Source: CAD feature listing. Evaluate the final solid. Frame: model axes, mm. Face numbers are marked on the shaded views. A direction names the side the tool comes from. Round coordinates to 2 decimals unless told otherwise and drop trailing zeros. Order: outer loops, then holes, each group sorted by start corner. A loop starts at its lowest first (then second) coordinate and runs counter-clockwise, first axis right, second up. Notation, with made-up numbers: (-37.75, -12) - (10.25, -12) arc R22 cw to (10.25, 8) - close; hole circle Ø2 at (-39.75, 34). An arc over 180 degrees is marked (long way). Use one line per item in the form item = value. Start each with the question number.
Q1. Ray query, line 1 (Z direction, x = -6, y = -16); line 2 (Z direction, x = -4.5, y = -15.5); line 3 (X direction, y = -16.5, z = 16). Return the intervals inside material, ascending. Write a range as [from, to].
Q2. Draft query along Z for the marked faces 4, 5 and 6. Return one class per face: released by +Z, released by -Z, zero draft, split by the parting line, or undercut.
Q3. Cut plane B-B, the plane x = -11.5. Return the cut outline in (y, z), and give its area (3 significant figures).
Q4. Cut plane C-C, the plane z = 12. Return the cut outline in (x, y), and give its area (3 significant figures).
Q5. Cut plane D-D, the plane y = 6. Return the cut outline in (x, z).
Q6. Cut plane A-A, the plane y = -10. Return the cut outline in (x, z).
Q7. Set-up query: the marked faces 1, 2 and 3. Return all of +Z, -Z, +X, -X, +Y, -Y with unobstructed straight access to the full face (end or side cutting, diameter ignored); none if empty.
Q8. Pin query (flat end, axial travel): pin 1 Ø1 at (y, z) = (-0.5, -10.5) entering from +X; pin 2 Ø1.5 at (y, z) = (-0.5, -18) entering from +X; pin 3 Ø1.5 at (x, y) = (-12.5, 5) entering from +Z; pin 4 Ø3 at (x, y) = (-14.5, -11) entering from +Z. Return the tip coordinate at first contact, or that it passes through.
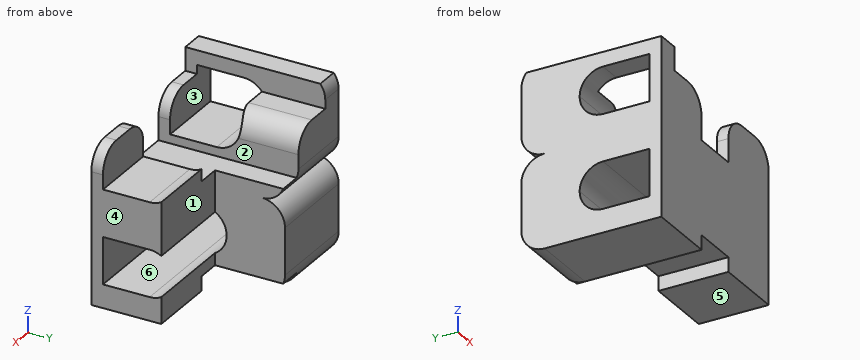
from build123d import *

# Parameters (mm, degrees)
F3_DEPTH = 25
F4_DEPTH = 25
F2_W     = 5
F2_H     = 5
F2_W_2   = 10
F2_H_2   = 20
F5_DEPTH = 25


with BuildPart() as f3:
    # F0 (on Top) → F3 (new body, symmetric)
    with BuildSketch(Plane.XY):
        Polygon((0, 20), (-20, 20), (-20, -20), (20, -20), (20, -5), (0, -5), align=None)
    extrude(amount=F3_DEPTH, both=True)

    # F1 (on Right) → F4 (intersect, symmetric)
    with BuildSketch(Plane.YZ):
        with BuildLine():
            Line((5, 20), (-20, 20))
            Line((-20, 20), (-20, -20))
            Line((-20, -20), (5, -20))
            ThreePointArc((5, -20), (8.535534, -18.535534), (10, -15))
            Line((10, -15), (10, -5))
            ThreePointArc((10, -5), (8.535534, -1.464466), (5, 0))
            ThreePointArc((5, 0), (8.535534, 1.464466), (10, 5))
            Line((10, 5), (10, 15))
            ThreePointArc((10, 15), (8.535534, 18.535534), (5, 20))
        make_face()
        with BuildLine():
            Line((-17.5, -5), (-7.5, -5))
            ThreePointArc((-7.5, -5), (-3.964466, -6.464466), (-2.5, -10))
            ThreePointArc((-2.5, -10), (-3.964466, -13.535534), (-7.5, -15))
            Line((-7.5, -15), (-17.5, -15))
            Line((-17.5, -15), (-17.5, -5))
        make_face(mode=Mode.SUBTRACT)
        with BuildLine():
            Line((-17.5, 15), (-7.5, 15))
            ThreePointArc((-7.5, 15), (-3.964466, 13.535534), (-2.5, 10))
            ThreePointArc((-2.5, 10), (-3.964466, 6.464466), (-7.5, 5))
            Line((-7.5, 5), (-17.5, 5))
            Line((-17.5, 5), (-17.5, 15))
        make_face(mode=Mode.SUBTRACT)
    extrude(amount=F4_DEPTH, both=True, mode=Mode.INTERSECT)

    # F2 (on Front) → F5 (intersect, symmetric)
    with BuildSketch(Plane.XZ):
        with Locations((-17.5, 15.590909)):
            Rectangle(F2_W, F2_H)
        with BuildLine():
            Line((-15, 13.090909), (-20, 13.090909))
            Line((-20, 13.090909), (-20, -21.909091))
            Line((-20, -21.909091), (-5, -21.909091))
            Line((-5, -21.909091), (-5, -16.909091))
            Line((-5, -16.909091), (-5, 3.090909))
            Line((-5, 3.090909), (-5, 8.090909))
            ThreePointArc((-5, 8.090909), (-6.464466, 11.626443), (-10, 13.090909))
            Line((-10, 13.090909), (-15, 13.090909))
        make_face()
        with Locations((0, -6.909091)):
            Rectangle(F2_W_2, F2_H_2)
        with BuildLine():
            Line((5, 3.090909), (5, -16.909091))
            Line((5, -16.909091), (5, -21.909091))
            Line((5, -21.909091), (20, -21.909091))
            Line((20, -21.909091), (20, 8.090909))
            ThreePointArc((20, 8.090909), (18.535534, 11.626443), (15, 13.090909))
            Line((15, 13.090909), (10, 13.090909))
            ThreePointArc((10, 13.090909), (6.464466, 11.626443), (5, 8.090909))
            Line((5, 8.090909), (5, 3.090909))
        make_face()
    extrude(amount=F5_DEPTH, both=True, mode=Mode.INTERSECT)


solid = f3.part
Completed:
q1.line_1 = [-20, -15], [-5, 5]
q1.line_2 = [-16.91, -15], [-5, 3.09]
q1.line_3 = [-20, -15]
q2.face_4 = zero draft
q2.face_5 = released by -Z
q2.face_6 = undercut
q3.outline = (-20, -20) - (5, -20) arc R5 ccw to (10, -15) - (10, -5) arc R5 ccw to (5, 0) arc R5 ccw to (10, 5) - (10, 13.09) - (-3.57, 13.09) arc R5 cw to (-7.5, 5) - (-17.5, 5) - (-17.5, 13.09) - (-20, 13.09) - close; hole (-17.5, -15) - (-7.5, -15) arc R5 ccw to (-7.5, -5) - (-17.5, -5) - close
q3.area = 722 mm2
q4.outline = (-20, -20) - (-6.88, -20) - (-6.88, -17.5) - (-20, -17.5) - close; (-20, -2.92) - (-6.88, -2.92) - (-6.88, 10) - (-20, 10) - close; (6.88, -20) - (18.12, -20) - (18.12, -17.5) - (6.88, -17.5) - close
q4.area = 230 mm2
q5.outline = (-20, -19.9) - (-5, -19.9) - (-5, -16.91) - (0, -16.91) - (0, -0.1) - (-20, -0.1) - close; (-20, 0.1) - (0, 0.1) - (0, 3.09) - (-5, 3.09) - (-5, 8.09) arc R5 ccw to (-10, 13.09) - (-15, 13.09) - (-15, 18.09) - (-20, 18.09) - close
q6.outline = (-20, -20) - (-5, -20) - (-5, -16.91) - (5, -16.91) - (5, -20) - (20, -20) - (20, -15) - (-20, -15) - close; (-20, -5) - (20, -5) - (20, 5) - (5, 5) - (5, 3.09) - (-5, 3.09) - (-5, 5) - (-20, 5) - close; (-20, 15) - (-15, 15) - (-15, 18.09) - (-20, 18.09) - close
q7.face_1 = +Z, -Z, +X, +Y
q7.face_2 = +Z, +Y, -Y
q7.face_3 = +X, -X
q8.pin_1 = 0
q8.pin_2 = -5
q8.pin_3 = 13.09
q8.pin_4 = 18.09
